from build123d import *

# Parameters (mm, degrees)
EXTRUIR1_DEPTH = 2


with BuildPart() as part:
    # Croquis1 → Extruir1 (new body)
    with BuildSketch(Plane.XY):
        with BuildLine():
            Line((200.095995896, 161.842834793), (200.095995896, 214.210663326))
            ThreePointArc((200.095995896, 214.210663326), (199.597250288, 216.26978044), (198.211567768, 217.872463947))
            Line((198.211567768, 217.872463947), (190.769475027, 223.188244475))
            ThreePointArc((190.769475027, 223.188244475), (189.527201595, 223.811773643), (188.153903155, 224.026443855))
            Line((188.153903155, 224.026443855), (164.038088636, 224.026443855))
            ThreePointArc((164.038088636, 224.026443855), (162.664790197, 223.811773643), (161.422516764, 223.188244475))
            Line((161.422516764, 223.188244475), (153.980424024, 217.872463947))
            ThreePointArc((153.980424024, 217.872463947), (152.594741504, 216.26978044), (152.095995896, 214.210663326))
            Line((152.095995896, 214.210663326), (152.095995896, 161.842834793))
            ThreePointArc((152.095995896, 161.842834793), (152.594741504, 159.783717679), (153.980424024, 158.181034173))
            Line((153.980424024, 158.181034173), (161.422516764, 152.865253644))
            ThreePointArc((161.422516764, 152.865253644), (162.664790197, 152.241724476), (164.038088636, 152.027054264))
            Line((164.038088636, 152.027054264), (188.153903155, 152.027054264))
            ThreePointArc((188.153903155, 152.027054264), (189.527201595, 152.241724476), (190.769475027, 152.865253644))
            Line((190.769475027, 152.865253644), (198.211567768, 158.181034173))
            ThreePointArc((198.211567768, 158.181034173), (199.597250288, 159.783717679), (200.095995896, 161.842834793))
        make_face()
        with BuildLine():
            Line((164.095995896, 158.027054265), (188.095995896, 158.027054265))
            ThreePointArc((188.095995896, 158.027054265), (189.595995896, 156.527054264), (188.095995896, 155.027054265))
            Line((188.095995896, 155.027054265), (164.095995896, 155.027054265))
            ThreePointArc((164.095995896, 155.027054265), (162.595995896, 156.527054264), (164.095995896, 158.027054265))
        make_face(mode=Mode.SUBTRACT)
        with BuildLine():
            Line((164.095995896, 221.027054265), (188.095995896, 221.027054265))
            ThreePointArc((188.095995896, 221.027054265), (189.595995896, 219.527054264), (188.095995896, 218.027054265))
            Line((188.095995896, 218.027054265), (164.095995896, 218.027054265))
            ThreePointArc((164.095995896, 218.027054265), (162.595995896, 219.527054264), (164.095995896, 221.027054265))
        make_face(mode=Mode.SUBTRACT)
    extrude(amount=EXTRUIR1_DEPTH)


solid = part.part
Could you check a few things on this model? Use its own coordinates, in mm. A direction names the side the tool comes from. Round coordinates to 2 decimals unless told otherwise and drop trailing zeros. Order: outer loops, then holes, each group sorted by start corner. A loop starts at its lowest first (then second) coordinate and runs counter-clockwise, first axis right, second up.
Q1. Imagine slicing it at A-A, the plane x = 186.5. List the corners of the cut face in (y, z) for me, then the cut area to 3 significant figures.
Geometry says:
outline: (152.03, 0) - (155.03, 0) - (155.03, 2) - (152.03, 2) - close; (158.03, 0) - (218.03, 0) - (218.03, 2) - (158.03, 2) - close; (221.03, 0) - (224.03, 0) - (224.03, 2) - (221.03, 2) - close
area: 132 mm2
Q2. Which directions (+Z, -Z, +X, -X, +Y, -Y) give clear straight access to the entire face, cutting with the end or side of a thin tool? Please do faces 1 (the face through (189.596, 156.56, 0.986)), 2 (the face through (152.61, 216.3, 0.99)).
Geometry says:
face 1: +Z, -Z
face 2: +Z, -Z, -X, +Y
Q3. Imagine slicing it at C-C, the plane y = 159. List the corners of the cut face in (x, z) for me.
Geometry says:
outline: (153.11, 0) - (199.08, 0) - (199.08, 2) - (153.11, 2) - close
Q4. Thinking about a two-plate mould opening in X: for faces 3 (the face through (189.546, 223.806, 0.986)), 4 (the face through (176, 224.026, 1)), 5 (the face through (176, 218.027, 1)), 6 (the face through (162.683, 223.818, 0.986)), which applies, released by +X, released by -X, zero draft, split by the parting line, or undercut?
Geometry says:
face 3: released by +X
face 4: zero draft
face 5: undercut
face 6: released by -X
Q5. Please list where these lines run through material, in increasing order: probe 1 along Y at (x, z) = (185, 1); probe 2 along X at (y, z) = (161.5, 0.5); probe 3 along Y at (x, z) = (192, 1.6).
Geometry says:
probe 1: y = 152.03 to 155.03, 158.03 to 218.03, 221.03 to 224.03
probe 2: x = 152.11 to 200.08
probe 3: y = 153.74 to 222.31
Q6. Imagine slicing it at D-D, the plane x = 157. List the corners of the cut face in (y, z) for me, then the cut area to 3 significant figures.
Geometry says:
outline: (156.02, 0) - (220.03, 0) - (220.03, 2) - (156.02, 2) - close
area: 128 mm2
Q7. Imagine slicing it at B-B, the plane z = 0.6. List the corners of the cut face in (x, y) for me, then the cut area to 3 significant figures.
Geometry says:
outline: (152.1, 161.84) arc R4.5 ccw to (153.98, 158.18) - (161.42, 152.87) arc R4.5 ccw to (164.04, 152.03) - (188.15, 152.03) arc R4.5 ccw to (190.77, 152.87) - (198.21, 158.18) arc R4.5 ccw to (200.1, 161.84) - (200.1, 214.21) arc R4.5 ccw to (198.21, 217.87) - (190.77, 223.19) arc R4.5 ccw to (188.15, 224.03) - (164.04, 224.03) arc R4.5 ccw to (161.42, 223.19) - (153.98, 217.87) arc R4.5 ccw to (152.1, 214.21) - close; hole (164.1, 155.03) - (188.1, 155.03) arc R1.5 ccw to (188.1, 158.03) - (164.1, 158.03) arc R1.5 ccw to start; hole (164.1, 218.03) - (188.1, 218.03) arc R1.5 ccw to (188.1, 221.03) - (164.1, 221.03) arc R1.5 ccw to start
area: 3,140 mm2
